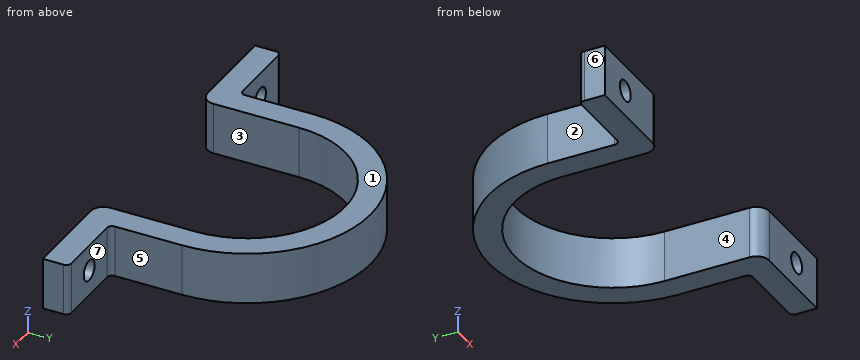
```python
from build123d import *

# Parameters (mm, degrees)
BOSS_EXTRUDE1_DEPTH = 20
SKETCH3_R           = 4
CUT_EXTRUDE2_DEPTH  = 20
FILLET3_R           = 2
FILLET4_R           = 5


with BuildPart() as part:
    # Sketch1 → Boss-Extrude1 (new body)
    with BuildSketch(Plane.XY):
        with BuildLine():
            Line((-38, -38), (-78, -38))
            Line((-78, -38), (-78, -28))
            Line((-78, -28), (-48, -28))
            Line((-48, -28), (-48, 0))
            ThreePointArc((-48, 0), (0, 48), (48, 0))
            Line((48, 0), (48, -28))
            Line((48, -28), (78, -28))
            Line((78, -28), (78, -38))
            Line((78, -38), (38, -38))
            Line((38, -38), (38, 0))
            ThreePointArc((38, 0), (0, 38), (-38, 0))
            Line((-38, 0), (-38, -38))
        make_face()
    extrude(amount=BOSS_EXTRUDE1_DEPTH)

    # Sketch3 → Cut-Extrude2 (cut)
    with BuildSketch(Plane(origin=(0, -28, 0), x_dir=(1, 0, 0), z_dir=(0, 1, 0))):
        with Locations((-63, -10)):
            Circle(SKETCH3_R)
        with Locations((63, -10)):
            Circle(SKETCH3_R)
    extrude(amount=-CUT_EXTRUDE2_DEPTH, mode=Mode.SUBTRACT)

    # Fillet3
    fillet3_edges = [part.edges().sort_by_distance(p)[0] for p in [
        (48, -28, 10),
        (78, -28, 10),
        (-78, -28, 10),
        (-48, -28, 10),
    ]]
    fillet(fillet3_edges, radius=FILLET3_R)

    # Fillet4
    fillet4_edges = [part.edges().sort_by_distance(p)[0] for p in [
        (38, -38, 10),
        (-38, -38, 10),
    ]]
    fillet(fillet4_edges, radius=FILLET4_R)


solid = part.part
```
Could you check a few things on this model? Use its own coordinates, in mm. Face numbers are marked on the shaded views. A direction names the side the tool comes from. Round coordinates to 2 decimals unless told otherwise and drop trailing zeros. Loops run counter-clockwise (first coordinate to the right, second up) from the corner with the lowest first, then second, coordinate; pieces in that order, holes last. Notation, with made-up numbers: (33, 12.25) - (65, 12.25) arc R31 ccw to (65, 38.25) - close; hole circle Ø4 at (-13.75, 81). An arc over 180 degrees is marked (long way). Use CSV: the item, a comma, the result in double quotes.
Item 1: If we mould it in two halves opening along X, with no side actions, what happens to the marked faces 4, 5, 6 and 7? For each: pulls with the +X half, pulls with the -X half, needs draft (parallel to the pull), parting line crosses it, or undercut.
Here are the results:
face 4,"undercut"
face 5,"pulls with the +X half"
face 6,"pulls with the -X half"
face 7,"needs draft"
Item 2: If we section it at D-D on x = 0: List the corners of the cut face in (y, z) for me.
Here are the results:
outline,"(38, 0) - (48, 0) - (48, 20) - (38, 20) - close"
Item 3: If we section it at B-B on y = -18: List the corners of the cut face in (x, z) for me.
Here are the results:
outline,"(-48, 0) - (-38, 0) - (-38, 20) - (-48, 20) - close; (38, 0) - (48, 0) - (48, 20) - (38, 20) - close"
Item 4: If we section it at C-C on z = 10: List the corners of the cut face in (x, y) for me, then the cut area to 3 significant figures.
Here are the results:
outline,"(-78, -38) - (-67, -38) - (-67, -28) - (-76, -28) arc R2 ccw to (-78, -30) - close; (-59, -38) - (-43, -38) arc R5 ccw to (-38, -33) - (-38, 0) arc R38 cw to (38, 0) - (38, -33) arc R5 ccw to (43, -38) - (59, -38) - (59, -28) - (50, -28) arc R2 cw to (48, -26) - (48, 0) arc R48 ccw to (-48, 0) - (-48, -26) arc R2 cw to (-50, -28) - (-59, -28) - close; (67, -38) - (78, -38) - (78, -30) arc R2 ccw to (76, -28) - (67, -28) - close"
area,"2,540 mm²"
Item 5: For the marked faces 1, 2 and 3, which set-ups out of +Z, -Z, +X, -X, +Y, -Y let a thin tool reach every point of the face, with its end or its side?
Here are the results:
face 1,"+Z, +X, -X, +Y, -Y"
face 2,"+Z, -Z, -X, +Y"
face 3,"+Z, -Z, -Y"
Item 6: I need wall thicknesses on L1, parallel to X at y = -31, z = 10; L2, parallel to Z at x = 63, y = -32.5; L3, parallel to X at y = -34.5, z = 10. Which ranges of each line are inside material? Lowest first, please. Write a range as [from, to].
Here are the results:
L1,"x = [-78, -67], [-59, -38], [38, 59], [67, 78]"
L2,"z = [0, 6], [14, 20]"
L3,"x = [-78, -67], [-59, -38.23], [38.23, 59], [67, 78]"
Item 7: If we section it at A-A on x = 63: List the corners of the cut face in (y, z) for me.
Here are the results:
outline,"(-38, 0) - (-28, 0) - (-28, 6) - (-38, 6) - close; (-38, 14) - (-28, 14) - (-28, 20) - (-38, 20) - close"
Item 8: Will these pins go through, and if not, where does the flat tip stop? pin 1 (7 mm diameter, centred on x = 63, z = 10, fed in from -Y); pin 2 (1.5 mm diameter, centred on y = 17.5, z = 2.5, fed in from -X); pin 3 (8 mm diameter, centred on y = 10.5, z = 15.5, fed in from -X); pin 4 (6 mm diameter, centred on x = 68, z = 8.5, fed in from +Y).
Here are the results:
pin 1,"passes through"
pin 2,"stops at x = -44.98"
pin 3,"stops at x = -47.56"
pin 4,"stops at y = -28"
